```python
from build123d import *

# Parameters (mm, degrees)
F0_R     = 1.1
F1_DEPTH = 1.5


with BuildPart() as f1:
    # F0 (on Top) → F1 (new body)
    with BuildSketch(Plane.XY):
        with BuildLine():
            ThreePointArc((17, 9), (16.707107, 9.707107), (16, 10))
            Line((16, 10), (-16, 10))
            ThreePointArc((-16, 10), (-16.707107, 9.707107), (-17, 9))
            Line((-17, 9), (-17, -9))
            ThreePointArc((-17, -9), (-16.707107, -9.707107), (-16, -10))
            Line((-16, -10), (16, -10))
            ThreePointArc((16, -10), (16.707107, -9.707107), (17, -9))
            Line((17, -9), (17, 9))
        make_face()
        with Locations((-13, -5)):
            Circle(F0_R, mode=Mode.SUBTRACT)
        with BuildLine():
            ThreePointArc((-5.5, -6.25), (-6.207107, -5.957107), (-6.5, -5.25))
            Line((-6.5, -5.25), (-6.5, -4.75))
            ThreePointArc((-6.5, -4.75), (-6.207107, -4.042893), (-5.5, -3.75))
            Line((-5.5, -3.75), (5.5, -3.75))
            ThreePointArc((5.5, -3.75), (6.207107, -4.042893), (6.5, -4.75))
            Line((6.5, -4.75), (6.5, -5.25))
            ThreePointArc((6.5, -5.25), (6.207107, -5.957107), (5.5, -6.25))
            Line((5.5, -6.25), (-5.5, -6.25))
        make_face(mode=Mode.SUBTRACT)
        with Locations((13, -5)):
            Circle(F0_R, mode=Mode.SUBTRACT)
        with Locations((-13, 5)):
            Circle(F0_R, mode=Mode.SUBTRACT)
        with BuildLine():
            ThreePointArc((-6.5, 5.25), (-6.207107, 5.957107), (-5.5, 6.25))
            Line((-5.5, 6.25), (5.5, 6.25))
            ThreePointArc((5.5, 6.25), (6.207107, 5.957107), (6.5, 5.25))
            Line((6.5, 5.25), (6.5, 4.75))
            ThreePointArc((6.5, 4.75), (6.207107, 4.042893), (5.5, 3.75))
            Line((5.5, 3.75), (-5.5, 3.75))
            ThreePointArc((-5.5, 3.75), (-6.207107, 4.042893), (-6.5, 4.75))
            Line((-6.5, 4.75), (-6.5, 5.25))
        make_face(mode=Mode.SUBTRACT)
        with Locations((13, 5)):
            Circle(F0_R, mode=Mode.SUBTRACT)
    extrude(amount=F1_DEPTH)


solid = f1.part
```
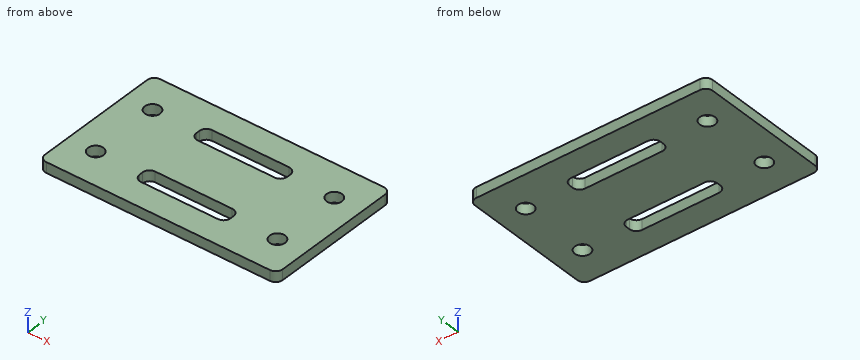
Input: part model. Units: mm. Frame: model coordinates. Coordinates: 2 decimals unless noted, no trailing zeros. Write each loop counter-clockwise with the first axis right and the second up, starting at its lowest first coordinate (ties: lowest second). Pieces come first, ordered by that corner, then holes.
1) Section C-C on x = -13. Output: boundary loops of the cut face in (y, z).
2) Section A-A on z = 0.3. Output: boundary loops of the cut face in (x, y).
3) Pin query (flat end, axial travel): pin 1 Ø2 at (x, y) = (-13, -5) entering from +Z. Return the tip coordinate at first contact, or that it passes through.
4) Material intervals for line 1 along Y through (x, z) = (4.5, 1.1); line 2 along Y through (x, z) = (13, 1.15); line 3 along X through (y, z) = (-4.5, 0.3), sorted ascending.
5) Section B-B on x = 4.5. Output: boundary loops of the cut face in (y, z).
Check result:
1. outline: (-10, 0) - (-6.1, 0) - (-6.1, 1.5) - (-10, 1.5) - close; (-3.9, 0) - (3.9, 0) - (3.9, 1.5) - (-3.9, 1.5) - close; (6.1, 0) - (10, 0) - (10, 1.5) - (6.1, 1.5) - close
2. outline: (-17, -9) arc R1 ccw to (-16, -10) - (16, -10) arc R1 ccw to (17, -9) - (17, 9) arc R1 ccw to (16, 10) - (-16, 10) arc R1 ccw to (-17, 9) - close; hole circle Ø2.2 at (-13, -5); hole circle Ø2.2 at (-13, 5); hole (-6.5, -5.25) arc R1 ccw to (-5.5, -6.25) - (5.5, -6.25) arc R1 ccw to (6.5, -5.25) - (6.5, -4.75) arc R1 ccw to (5.5, -3.75) - (-5.5, -3.75) arc R1 ccw to (-6.5, -4.75) - close; hole (-6.5, 4.75) arc R1 ccw to (-5.5, 3.75) - (5.5, 3.75) arc R1 ccw to (6.5, 4.75) - (6.5, 5.25) arc R1 ccw to (5.5, 6.25) - (-5.5, 6.25) arc R1 ccw to (-6.5, 5.25) - close; hole circle Ø2.2 at (13, -5); hole circle Ø2.2 at (13, 5)
3. pin 1: passes through
4. line 1: y = -10 to -6.25, -3.75 to 3.75, 6.25 to 10
4. line 2: y = -10 to -6.1, -3.9 to 3.9, 6.1 to 10
4. line 3: x = -17 to -13.98, -12.02 to -6.47, 6.47 to 12.02, 13.98 to 17
5. outline: (-10, 0) - (-6.25, 0) - (-6.25, 1.5) - (-10, 1.5) - close; (-3.75, 0) - (3.75, 0) - (3.75, 1.5) - (-3.75, 1.5) - close; (6.25, 0) - (10, 0) - (10, 1.5) - (6.25, 1.5) - close
